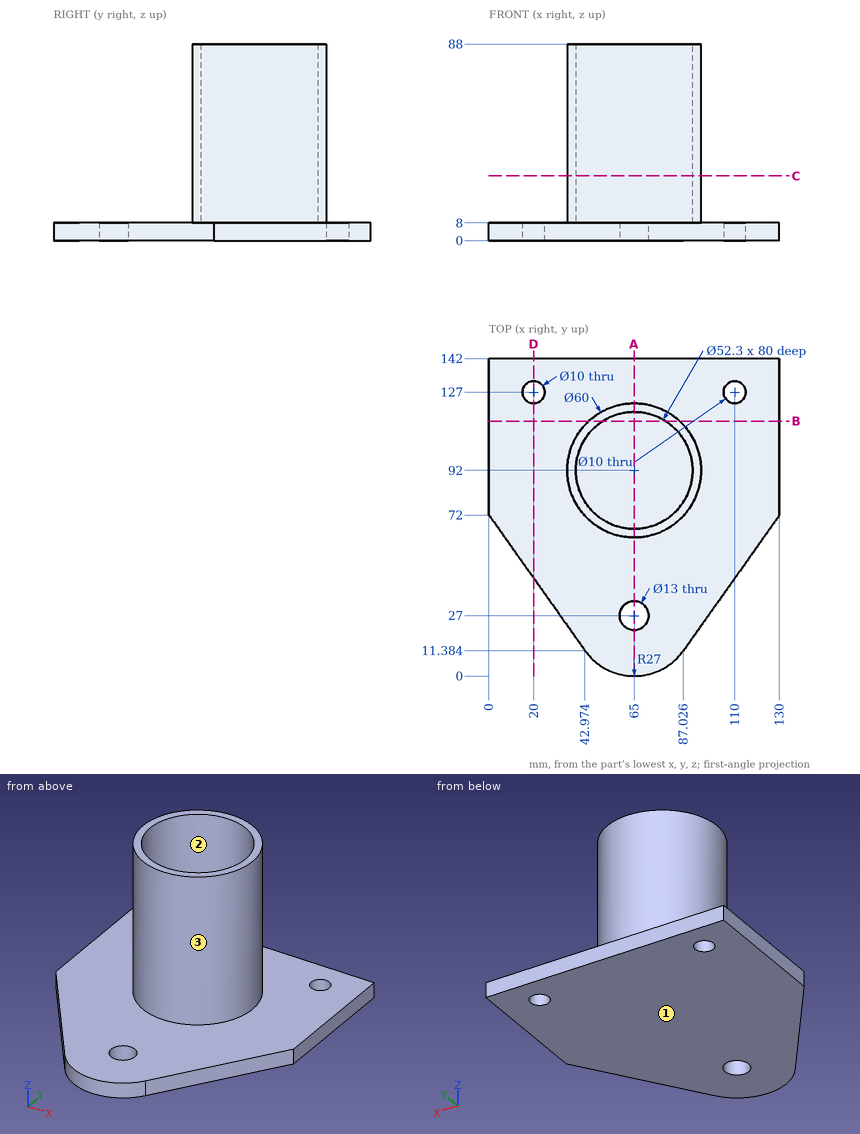
Geometry check sheet. Reference: drawing and pictorial views, mm from the part's lowest x, y, z. Round coordinates to 2 decimals unless told otherwise and drop trailing zeros. Order: outer loops, then holes, each group sorted by start corner. A loop starts at its lowest first (then second) coordinate and runs counter-clockwise, first axis right, second up. Notation, with made-up numbers: (-16, 67) - (36, 67) arc R9 ccw to (36, 75) - close; hole circle Ø11 at (57.25, 19.25). An arc over 180 degrees is marked (long way). Use a Markdown table: item, result. Add a question column.
1) Section check C-C (z = 29). Record the cut outline in (x, y), then the cut area to 3 significant figures.
2) Mould release check, pull along X, two halves, no side actions. Record for the marked faces 1, 2 and 3: released by +X, released by -X, zero draft, split by the parting line, or undercut.
3) Thickness scan on line 1 along Y through (x, z) = (65, 6.25); line 2 along Z through (x, y) = (103, 56); line 3 along Y through (x, z) = (77.5, 66). Record the ranges inside material, lowest first.
4) Section check B-B (y = 114). Record the cut outline in (x, z).
5) Gauge pin test, flat ends, axial feed: P1, Ø9, axis at x = 110, y = 127, coming from the +Z side; P2, Ø1, axis at x = 16.5, y = 118, coming from the +Z side; P3, Ø12, axis at x = 89.5, z = 23.5, coming from the -Y side; P4, Ø1.5, axis at y = 88.5, z = 29, coming from the +X side. Record the tip position at first contact, or that the pin passes through.
6) Section check D-D (x = 20). Record the cut outline in (y, z).
7) Section check A-A (x = 65). Record the cut outline in (y, z).
Established:
| question | item | result |
|---|---|---|
| 1 | outline | circle Ø60 at (65, 92); hole circle Ø52.3 at (65, 92) |
| 1 | area | 679 mm2 |
| 2 | face 1 | zero draft |
| 2 | face 2 | undercut |
| 2 | face 3 | split by the parting line |
| 3 | line 1 | 0 to 20.5, 33.5 to 142 |
| 3 | line 2 | 0 to 8 |
| 3 | line 3 | 64.73 to 69.03, 114.97 to 119.27 |
| 4 | outline | (0, 0) - (130, 0) - (130, 8) - (85.4, 8) - (85.4, 88) - (79.14, 88) - (79.14, 8) - (50.86, 8) - (50.86, 88) - (44.6, 88) - (44.6, 8) - (0, 8) - close |
| 5 | P1 | through |
| 5 | P2 | z = 8 |
| 5 | P3 | y = 68.38 |
| 5 | P4 | x = 94.87 |
| 6 | outline | (43.79, 0) - (122, 0) - (122, 8) - (43.79, 8) - close; (132, 0) - (142, 0) - (142, 8) - (132, 8) - close |
| 7 | outline | (0, 0) - (20.5, 0) - (20.5, 8) - (0, 8) - close; (33.5, 0) - (142, 0) - (142, 8) - (122, 8) - (122, 88) - (118.15, 88) - (118.15, 8) - (65.85, 8) - (65.85, 88) - (62, 88) - (62, 8) - (33.5, 8) - close |
